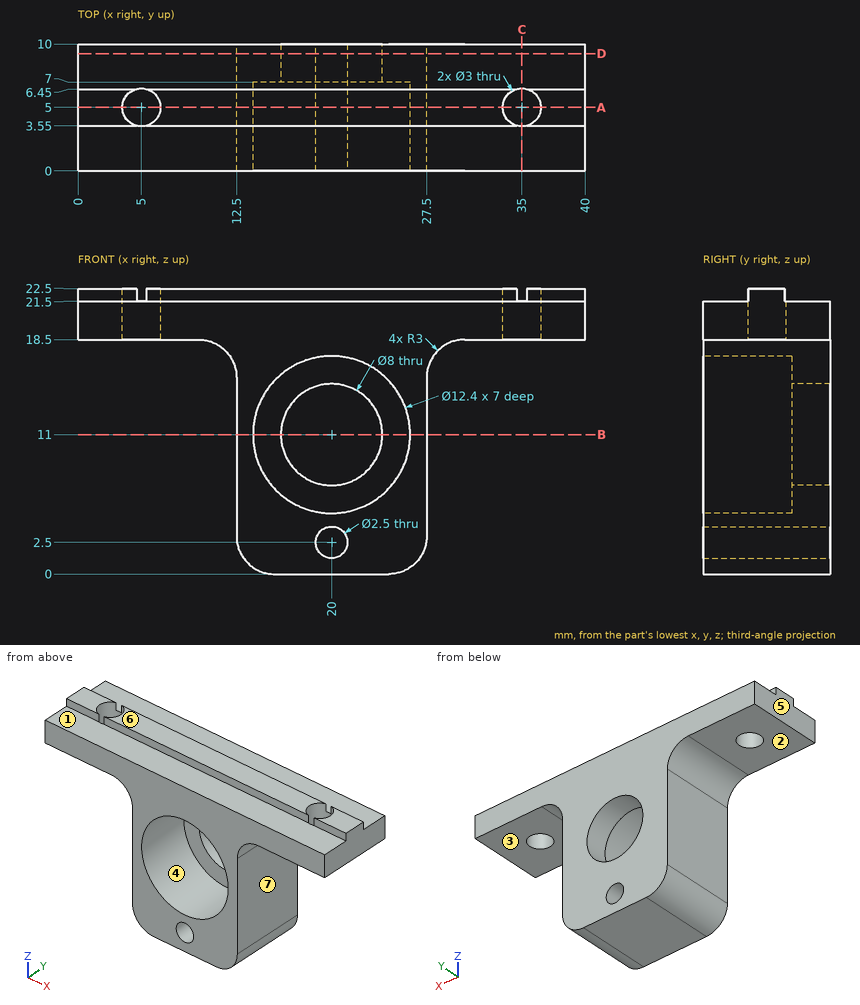
Verification items for this drawing (mm, ordinates from the low corner). A direction names the side the tool comes from. Coordinates: 2 decimals unless noted, no trailing zeros. Order: outer loops, then holes, each group sorted by start corner. A loop starts at its lowest first (then second) coordinate and runs counter-clockwise, first axis right, second up. Notation, with made-up numbers: M 46,55 L 75,55 A16 ccw 75,76 Z; hole C 52,-20.75 d11. An arc over 180 degrees is marked long. Answer as a JSON object with one key per item and string values.
Q1. Cross-section at A-A on y = 5. Record the cut outline in (x, z).
Results are:
{"outline": "M 0,18.5 L 3.5,18.5 L 3.5,22.5 L 0,22.5 Z; M 6.5,18.5 L 9.5,18.5 A3 cw 12.5,15.5 L 12.5,3 A3 ccw 15.5,0 L 24.5,0 A3 ccw 27.5,3 L 27.5,15.5 A3 cw 30.5,18.5 L 33.5,18.5 L 33.5,22.5 L 6.5,22.5 Z; M 36.5,18.5 L 40,18.5 L 40,22.5 L 36.5,22.5 Z; hole C 20,11 d12.4; hole C 20,2.5 d2.5"}
Q2. Tool access check on the marked faces 1, 2 and 3. Record the directions out of +Z, -Z, +X, -X, +Y, -Y that give a thin tool (end or side, any length) a straight path to the whole face; none if there is none.
Results are:
{"face 1": "+Z, +X, -X, -Y", "face 2": "-Z, -X, +Y, -Y", "face 3": "-Z, +X, +Y, -Y"}
Q3. Depth check by flat-ended pin: pin 1 Ø1.5 at (y, z) = (7.5, 6.5) entering from -X; pin 2 Ø1.1 at (x, y) = (25.5, 9) entering from +Z; pin 3 Ø10 at (x, z) = (19.5, 10.5) entering from -Y. Enter the tip coordinate at first touch or a pass-through.
Results are:
{"pin 1": "stops at x = 12.5", "pin 2": "stops at z = 21.5", "pin 3": "stops at y = 7"}
Q4. Cross-section at C-C on x = 35. Record the cut outline in (y, z), and give its area (3 significant figures).
Results are:
{"outline": "M 0,18.5 L 3.5,18.5 L 3.5,21.5 L 0,21.5 Z; M 6.5,18.5 L 10,18.5 L 10,21.5 L 6.5,21.5 Z", "area": "21.0 mm²"}
Q5. Cross-section at D-D on y = 9.25. Record the cut outline in (x, z).
Results are:
{"outline": "M 0,18.5 L 9.5,18.5 A3 cw 12.5,15.5 L 12.5,3 A3 ccw 15.5,0 L 24.5,0 A3 ccw 27.5,3 L 27.5,15.5 A3 cw 30.5,18.5 L 40,18.5 L 40,21.5 L 0,21.5 Z; hole C 20,11 d8; hole C 20,2.5 d2.5"}
Q6. Scan lines: line 1 (Z direction, x = 20, y = 8.1); line 2 (Z direction, x = 20, y = 5.75); line 3 (Y direction, x = 5, z = 20.45). Record each from-to range of solid material in increasing order.
Results are:
{"line 1": "z = 0 to 1.25, 3.75 to 7, 15 to 21.5", "line 2": "z = 0 to 1.25, 3.75 to 4.8, 17.2 to 22.5", "line 3": "y = 0 to 3.5, 6.5 to 10"}
Q7. Release check for a two-part mould opening along X. For the marked faces 4, 5, 6 and 7 record: released by +X, released by -X, zero draft, split by the parting line, or undercut.
Results are:
{"face 4": "undercut", "face 5": "released by -X", "face 6": "zero draft", "face 7": "released by +X"}
Q8. Cross-section at B-B on z = 11. Record the cut outline in (x, y), and give its area (3 significant figures).
Results are:
{"outline": "M 12.5,0 L 13.8,0 L 13.8,7 L 16,7 L 16,10 L 12.5,10 Z; M 24,7 L 26.2,7 L 26.2,0 L 27.5,0 L 27.5,10 L 24,10 Z", "area": "39.2 mm²"}
